Check sheet for the modelled part. Datum: model origin and axes. Units: mm. Face numbers are marked on the shaded views. A direction names the side the tool comes from. Coordinates: 2 decimals unless noted, no trailing zeros. Write each loop counter-clockwise with the first axis right and the second up, starting at its lowest first coordinate (ties: lowest second). Pieces come first, ordered by that corner, then holes. Notation, with made-up numbers: M -38.5,-15 L -16.5,-15 A17 cw -16.5,5 Z; hole C 0,76.5 d6. An arc over 180 degrees is marked long. Answer as CSV lines item,"result". Start each with the question number.
1) Access from +Z, -Z, +X, -X, +Y, -Y to the whole of each face (thin tool, end or side, straight path). Record for the marked faces 1, 2, 3 and 4.
2) Section check B-B (y = 10.5). Record the cut outline in (x, z).
3) Material ranges on L1, parallel to Z at x = 84, y = 22.45; L2, parallel to Z at x = 118.5, y = 4.5; L3, parallel to X at y = 3, z = 41, recorded low to high. Write a range as [from, to].
4) Section check C-C (z = 5). Record the cut outline in (x, y).
5) Draft check along Y on the marked faces 5, 6, 7 and 8. Enter one of: +Y half, -Y half, draft (parallel to the pull), parting line (faces both ways), or undercut.
6) Go/stop test with flat-tipped pins: pin 1 Ø24.5 at (x, y) = (37, 30.5) entering from -Z; pin 2 Ø15.5 at (x, z) = (84, 28) entering from +Y; pin 3 Ø14.5 at (x, y) = (72.5, 27.5) entering from +Z; pin 4 Ø12 at (y, z) = (29, 26) entering from +X. Record where each tip stops, or that it passes through.
7) Section check A-A (z = 28). Record the cut outline in (x, y), and give its area (3 significant figures).
8) Section check D-D (x = 84). Record the cut outline in (y, z), and give its area (3 significant figures).
from build123d import *

# Parameters (mm, degrees)
BOSS_EXTRUDE1_DEPTH = 56
FILLET1_R           = 10
SKETCH2_R           = 4
CUT_EXTRUDE1_DEPTH  = 56
SKETCH4_R           = 11
SKETCH4_R_2         = 6
BOSS_EXTRUDE2_DEPTH = 10
CUT_EXTRUDE2_START  = -34
SKETCH5_R           = 6
CUT_EXTRUDE2_DEPTH  = 34
SKETCH6_R           = 14
SKETCH6_R_2         = 8
BOSS_EXTRUDE3_DEPTH = 56
BOSS_EXTRUDE4_START = -7
BOSS_EXTRUDE4_DEPTH = 7
BOSS_EXTRUDE5_DEPTH = 7


with BuildPart() as part:
    # Sketch1 → Boss-Extrude1 (new body)
    with BuildSketch(Plane.XY):
        with BuildLine():
            Line((0, 0), (70, 0))
            ThreePointArc((70, 0), (84, 14), (98, 0))
            Line((98, 0), (126, 0))
            Line((126, 0), (126, 8))
            Line((126, 8), (103.416487839, 8))
            ThreePointArc((103.416487839, 8), (84, 21), (64.583512161, 8))
            Line((64.583512161, 8), (0, 8))
            Line((0, 8), (0, 0))
        make_face()
    extrude(amount=BOSS_EXTRUDE1_DEPTH)

    # Fillet1
    fillet1_edges = [part.edges().sort_by_distance(p)[0] for p in [
        (0, 4, 0),
        (126, 4, 56),
        (0, 4, 56),
        (126, 4, 0),
    ]]
    fillet(fillet1_edges, radius=FILLET1_R)

    # Sketch2 → Cut-Extrude1 (cut)
    with BuildSketch(Plane(origin=(0, 8, 0), x_dir=(1, 0, 0), z_dir=(0, 1, 0))):
        with Locations(Location((10, -15, 0), (0, 0, 270))):
            Circle(SKETCH2_R)
        with Locations(Location((10, -41, 0), (0, 0, 270))):
            Circle(SKETCH2_R)
        with Locations(Location((116, -15, 0), (0, 0, 270))):
            Circle(SKETCH2_R)
        with Locations(Location((116, -41, 0), (0, 0, 270))):
            Circle(SKETCH2_R)
    extrude(amount=-CUT_EXTRUDE1_DEPTH, mode=Mode.SUBTRACT)

    # Sketch4 → Boss-Extrude2 (add)
    with BuildSketch(Plane(origin=(0, 14, 0), x_dir=(-1, 0, 0), z_dir=(0, -1, 0))):
        with Locations(Location((-84, -28, 0), (0, 0, 90))):
            Circle(SKETCH4_R)
        with Locations(Location((-84, -28, 0), (0, 0, 90))):
            Circle(SKETCH4_R_2, mode=Mode.SUBTRACT)
    extrude(amount=-BOSS_EXTRUDE2_DEPTH)

    # Sketch5 → Cut-Extrude2 (cut)
    with BuildSketch(Plane(origin=(0, 24, 0), x_dir=(1, 0, 0), z_dir=(0, 1, 0)).offset(CUT_EXTRUDE2_START)):
        with Locations(Location((84, -28, 0), (0, 0, 90))):
            Circle(SKETCH5_R)
    extrude(amount=CUT_EXTRUDE2_DEPTH, mode=Mode.SUBTRACT)



with BuildPart() as body_2:
    # Sketch6 → Boss-Extrude3 (new body)
    with BuildSketch(Plane.XY):
        with Locations((31, 45)):
            Circle(SKETCH6_R)
        with Locations((31, 45)):
            Circle(SKETCH6_R_2, mode=Mode.SUBTRACT)
    extrude(amount=BOSS_EXTRUDE3_DEPTH)


with BuildPart() as part_1:
    add(part.part)

    add(body_2.part)  # Boss-Extrude4 merges body 2
    # Sketch7 → Boss-Extrude4 (add)
    with BuildSketch(Plane.XY.offset(54).offset(BOSS_EXTRUDE4_START)):
        with BuildLine():
            Line((17, 45), (17, 8))
            Line((17, 8), (64.583512161, 8))
            ThreePointArc((64.583512161, 8), (78.026449954, 20.132478731), (95.911075968, 17.295267251))
            Line((95.911075968, 17.295267251), (38.940717312, 56.530178167))
            ThreePointArc((38.940717312, 56.530178167), (37.512678314, 32.607057606), (17, 45))
        make_face()
    extrude(amount=BOSS_EXTRUDE4_DEPTH)

    # Sketch8 → Boss-Extrude5 (add)
    with BuildSketch(Plane(origin=(0, 0, 2), x_dir=(-1, 0, 0), z_dir=(0, 0, -1))):
        with BuildLine():
            Line((-17, 45), (-17, 8))
            Line((-17, 8), (-64.583512161, 8))
            ThreePointArc((-64.583512161, 8), (-78.026449954, 20.132478731), (-95.911075968, 17.295267251))
            Line((-95.911075968, 17.295267251), (-38.940717312, 56.530178167))
            ThreePointArc((-38.940717312, 56.530178167), (-37.512678314, 32.607057606), (-17, 45))
        make_face()
    extrude(amount=-BOSS_EXTRUDE5_DEPTH)


solid = part_1.part
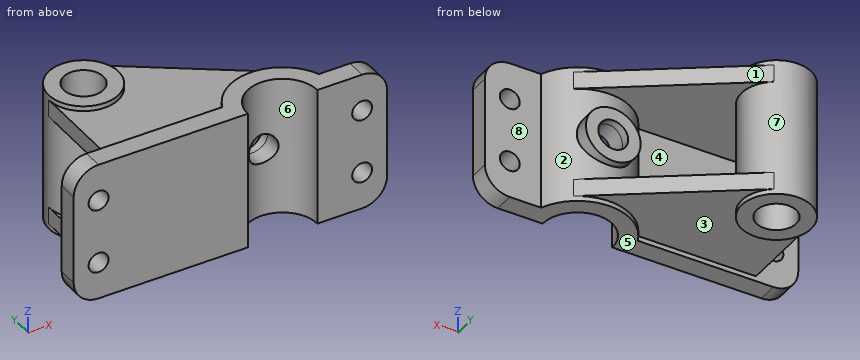
Results found:
1,face 1,"+Z, +X, +Y"
1,face 2,"+Y"
1,face 3,"-Z"
1,face 4,"-X"
2,outline,"M 17,2 L 65.81,2 L 65.81,0 L 74.74,0 L 74.74,56 L 65.81,56 L 65.81,54 L 17,54 L 17,47 L 65.81,47 L 65.81,9 L 17,9 Z; M 93.26,0 L 102.19,0 L 102.19,56 L 93.26,56 Z"
3,L1,"z = [2, 9], [17, 22], [34, 39], [47, 54]"
3,L2,"z = [0.32, 11.88], [18.12, 37.88], [44.12, 55.68]"
3,L3,"x = [0, 6], [14, 70.33], [97.67, 112], [120, 126]"
4,outline,"M 1.34,0 L 70,0 A14 cw 98,0 L 124.66,0 L 124.66,8 L 103.42,8 A21 ccw 95.91,17.3 L 38.94,56.53 A14 ccw 17,45 L 17,8 L 1.34,8 Z; hole C 31,45 d16"
5,face 5,"draft"
5,face 6,"-Y half"
5,face 7,"undercut"
5,face 8,"+Y half"
6,pin 1,"stops at z = 0"
6,pin 2,"stops at y = 24"
6,pin 3,"stops at z = 54"
6,pin 4,"stops at x = 95"
7,outline,"M 0,0 L 70,0 A14 cw 78,12.65 L 78,24 L 73,24 L 73,17.89 A21 ccw 64.58,8 L 0,8 Z; C 31,45 d28; M 90,12.65 A14 cw 98,0 L 126,0 L 126,8 L 103.42,8 A21 ccw 95,17.89 L 95,24 L 90,24 Z; hole C 31,45 d16"
7,area,"1,440 mm2"
8,outline,"M 14,0 L 21,0 L 21,2 L 25.5,2 L 25.5,9 L 21,9 L 21,17 L 24,17 L 24,22 L 14,22 Z; M 14,34 L 24,34 L 24,39 L 21,39 L 21,47 L 25.5,47 L 25.5,54 L 21,54 L 21,56 L 14,56 Z"
8,area,"401 mm2"
